Could you check a few things on this model? Use its own coordinates, in mm. Give positions to 0.01 mm unless a question says otherwise; leave off trailing zeros. Put each result on its own line as item: value.
```python
from build123d import *

# Parameters (mm, degrees)
SKETCH1_R           = 12.7
BOSS_EXTRUDE1_DEPTH = 6.35
FILLET1_R           = 1.5875
FILLET2_R           = 3.175


with BuildPart() as part:
    # Sketch1 → Boss-Extrude1 (new, symmetric)
    with BuildSketch(Plane.XY):
        Polygon((-9.43506227631135, 19.870822827505833), (-21.92616850087544, 1.7644077961790767), (-12.491106224564081, -18.10641503132676), (9.43506227631137, -19.870822827505812), (21.926168500875455, -1.764407796179048), (12.491106224564096, 18.10641503132678), align=None)
        Circle(SKETCH1_R, mode=Mode.SUBTRACT)
    extrude(amount=BOSS_EXTRUDE1_DEPTH, both=True)

    # Fillet1
    fillet1_edges = [part.edges().sort_by_distance(p)[0] for p in [
        (-17.208637362719763, -8.17100361757384, 6.35),
        (-1.5280219741263554, -18.988618929416283, 6.35),
        (15.680615388593413, -10.81761531184243, 6.35),
        (17.208637362719777, 8.171003617573865, 6.35),
        (1.5280219741263732, 18.988618929416305, 6.35),
        (17.208637362719777, 8.171003617573865, -6.35),
        (15.680615388593413, -10.81761531184243, -6.35),
        (-1.5280219741263554, -18.988618929416283, -6.35),
        (-17.208637362719763, -8.17100361757384, -6.35),
        (-15.680615388593395, 10.817615311842456, -6.35),
        (1.5280219741263732, 18.988618929416305, -6.35),
        (-15.680615388593395, 10.817615311842456, 6.35),
    ]]
    fillet(fillet1_edges, radius=FILLET1_R)

    # Fillet2
    # the kernel refuses this fillet: 3.175 mm, written as the material it takes off along each edge
    with BuildSketch(Plane(origin=(-7.862551896926124, 16.559019022921532, -6.35), x_dir=(-0.8231294167240627, 0.5678538221439602, 0), z_dir=(-0.5678538221439602, -0.8231294167240627, 0))) as fillet2_piece_1:
        with BuildLine():
            CenterArc((1.5875, -1.5875), 1.5875, 0, 90)
            Line((3.175, -1.5875), (3.175, 0))
            Line((3.175, 0), (1.5875, 0))
        make_face()
    revolve(axis=Axis((-7.862551896926124, 16.559019022921532, -6.35), (0, 0, -1)), revolution_arc=59.999999999999986, mode=Mode.SUBTRACT)
    with BuildSketch(Plane(origin=(10.409255187136749, 15.088679192772318, -6.35), x_dir=(0.08021112725072843, 0.996777896557286, 0), z_dir=(-0.996777896557286, 0.08021112725072843, 0))) as fillet2_piece_2:
        with BuildLine():
            CenterArc((1.5875, -1.5875), 1.5875, 0, 90)
            Line((3.175, -1.5875), (3.175, 0))
            Line((3.175, 0), (1.5875, 0))
        make_face()
    revolve(axis=Axis((10.409255187136749, 15.088679192772318, -6.35), (0, 0, -1)), revolution_arc=59.99999999999997, mode=Mode.SUBTRACT)
    with BuildSketch(Plane(origin=(-18.271807084062868, 1.470339830149234, -6.35), x_dir=(-0.9033405439747911, -0.4289240744133263, 0), z_dir=(0.4289240744133263, -0.9033405439747911, 0))) as fillet2_piece_3:
        with BuildLine():
            CenterArc((1.5875, -1.5875), 1.5875, 0, 90)
            Line((3.175, -1.5875), (3.175, 0))
            Line((3.175, 0), (1.5875, 0))
        make_face()
    revolve(axis=Axis((-18.271807084062868, 1.470339830149234, -6.35), (0, 0, -1)), revolution_arc=60.000000000000036, mode=Mode.SUBTRACT)
    with BuildSketch(Plane(origin=(18.27180708406288, -1.4703398301492088, -6.35), x_dir=(0.903340543974791, 0.4289240744133264, 0), z_dir=(-0.4289240744133264, 0.903340543974791, 0))) as fillet2_piece_4:
        with BuildLine():
            CenterArc((1.5875, -1.5875), 1.5875, 0, 90)
            Line((3.175, -1.5875), (3.175, 0))
            Line((3.175, 0), (1.5875, 0))
        make_face()
    revolve(axis=Axis((18.27180708406288, -1.4703398301492088, -6.35), (0, 0, -1)), revolution_arc=60.00000000000001, mode=Mode.SUBTRACT)
    with BuildSketch(Plane(origin=(-10.40925518713673, -15.0886791927723, -6.35), x_dir=(-0.0802111272507284, -0.996777896557286, 0), z_dir=(0.996777896557286, -0.0802111272507284, 0))) as fillet2_piece_5:
        with BuildLine():
            CenterArc((1.5875, -1.5875), 1.5875, 0, 90)
            Line((3.175, -1.5875), (3.175, 0))
            Line((3.175, 0), (1.5875, 0))
        make_face()
    revolve(axis=Axis((-10.40925518713673, -15.0886791927723, -6.35), (0, 0, -1)), revolution_arc=59.99999999999997, mode=Mode.SUBTRACT)
    with BuildSketch(Plane(origin=(7.862551896926148, -16.559019022921508, -6.35), x_dir=(0.823129416724063, -0.5678538221439597, 0), z_dir=(0.5678538221439597, 0.823129416724063, 0))) as fillet2_piece_6:
        with BuildLine():
            CenterArc((1.5875, -1.5875), 1.5875, 0, 90)
            Line((3.175, -1.5875), (3.175, 0))
            Line((3.175, 0), (1.5875, 0))
        make_face()
    revolve(axis=Axis((7.862551896926148, -16.559019022921508, -6.35), (0, 0, -1)), revolution_arc=60.00000000000002, mode=Mode.SUBTRACT)
    with BuildSketch(Plane(origin=(7.862551896926148, -16.559019022921508, 6.35), x_dir=(-0.0802111272507284, -0.996777896557286, 0), z_dir=(-0.996777896557286, 0.0802111272507284, 0))) as fillet2_piece_7:
        with BuildLine():
            CenterArc((1.5875, -1.5875), 1.5875, 0, 90)
            Line((3.175, -1.5875), (3.175, 0))
            Line((3.175, 0), (1.5875, 0))
        make_face()
    revolve(axis=Axis((7.862551896926148, -16.559019022921508, 6.35), (0, 0, 1)), revolution_arc=60.00000000000002, mode=Mode.SUBTRACT)
    with BuildSketch(Plane(origin=(-10.40925518713673, -15.0886791927723, 6.35), x_dir=(-0.9033405439747911, -0.4289240744133263, 0), z_dir=(-0.4289240744133263, 0.9033405439747911, 0))) as fillet2_piece_8:
        with BuildLine():
            CenterArc((1.5875, -1.5875), 1.5875, 0, 90)
            Line((3.175, -1.5875), (3.175, 0))
            Line((3.175, 0), (1.5875, 0))
        make_face()
    revolve(axis=Axis((-10.40925518713673, -15.0886791927723, 6.35), (0, 0, 1)), revolution_arc=59.99999999999997, mode=Mode.SUBTRACT)
    with BuildSketch(Plane(origin=(18.27180708406288, -1.4703398301492088, 6.35), x_dir=(0.823129416724063, -0.5678538221439597, 0), z_dir=(-0.5678538221439597, -0.823129416724063, 0))) as fillet2_piece_9:
        with BuildLine():
            CenterArc((1.5875, -1.5875), 1.5875, 0, 90)
            Line((3.175, -1.5875), (3.175, 0))
            Line((3.175, 0), (1.5875, 0))
        make_face()
    revolve(axis=Axis((18.27180708406288, -1.4703398301492088, 6.35), (0, 0, 1)), revolution_arc=60.00000000000001, mode=Mode.SUBTRACT)
    with BuildSketch(Plane(origin=(-18.271807084062868, 1.470339830149234, 6.35), x_dir=(-0.8231294167240627, 0.5678538221439602, 0), z_dir=(0.5678538221439602, 0.8231294167240627, 0))) as fillet2_piece_10:
        with BuildLine():
            CenterArc((1.5875, -1.5875), 1.5875, 0, 90)
            Line((3.175, -1.5875), (3.175, 0))
            Line((3.175, 0), (1.5875, 0))
        make_face()
    revolve(axis=Axis((-18.271807084062868, 1.470339830149234, 6.35), (0, 0, 1)), revolution_arc=60.000000000000036, mode=Mode.SUBTRACT)
    with BuildSketch(Plane(origin=(10.409255187136749, 15.088679192772318, 6.35), x_dir=(0.903340543974791, 0.4289240744133264, 0), z_dir=(0.4289240744133264, -0.903340543974791, 0))) as fillet2_piece_11:
        with BuildLine():
            CenterArc((1.5875, -1.5875), 1.5875, 0, 90)
            Line((3.175, -1.5875), (3.175, 0))
            Line((3.175, 0), (1.5875, 0))
        make_face()
    revolve(axis=Axis((10.409255187136749, 15.088679192772318, 6.35), (0, 0, 1)), revolution_arc=59.99999999999997, mode=Mode.SUBTRACT)
    with BuildSketch(Plane(origin=(-7.862551896926124, 16.559019022921532, 6.35), x_dir=(0.08021112725072843, 0.996777896557286, 0), z_dir=(0.996777896557286, -0.08021112725072843, 0))) as fillet2_piece_12:
        with BuildLine():
            CenterArc((1.5875, -1.5875), 1.5875, 0, 90)
            Line((3.175, -1.5875), (3.175, 0))
            Line((3.175, 0), (1.5875, 0))
        make_face()
    revolve(axis=Axis((-7.862551896926124, 16.559019022921532, 6.35), (0, 0, 1)), revolution_arc=59.999999999999986, mode=Mode.SUBTRACT)
    with BuildSketch(Plane(origin=(9.43506227631137, -19.870822827505812, -6.35), x_dir=(-0.9967778965572859, 0.08021112725072867, 0), z_dir=(0, 0, 1))) as fillet2_piece_13:
        with BuildLine():
            CenterArc((FILLET2_R * 0.57735026919, -FILLET2_R), FILLET2_R, 90.00000000000003, 60)
            Line((-FILLET2_R * 0.288675134595, -FILLET2_R * 0.5), (0, 0))
            Line((0, 0), (FILLET2_R * 0.57735026919, -3e-17))
        make_face()
    extrude(amount=12.7, mode=Mode.SUBTRACT)
    with BuildSketch(Plane(origin=(-12.491106224564081, -18.106415031326755, -6.35), x_dir=(-0.4289240744133256, 0.9033405439747914, 0), z_dir=(0, 0, 1))) as fillet2_piece_14:
        with BuildLine():
            CenterArc((FILLET2_R * 0.57735026919, -FILLET2_R), FILLET2_R, 90.00000000000006, 59.99999999999994)
            Line((-FILLET2_R * 0.288675134595, -FILLET2_R * 0.5), (0, 0))
            Line((0, 0), (FILLET2_R * 0.57735026919, -1.1e-16))
        make_face()
    extrude(amount=12.7, mode=Mode.SUBTRACT)
    with BuildSketch(Plane(origin=(-21.92616850087544, 1.764407796179075, -6.350000000000001), x_dir=(0.5678538221439581, 0.8231294167240641, 0), z_dir=(0, 0, 1))) as fillet2_piece_15:
        with BuildLine():
            CenterArc((FILLET2_R * 0.57735026919, -FILLET2_R), FILLET2_R, 89.99999999999986, 60.000000000000114)
            Line((-FILLET2_R * 0.288675134595, -FILLET2_R * 0.5), (0, 0))
            Line((0, 0), (FILLET2_R * 0.57735026919, 0))
        make_face()
    extrude(amount=12.700000000000001, mode=Mode.SUBTRACT)
    with BuildSketch(Plane(origin=(-9.43506227631135, 19.870822827505833, 6.35), x_dir=(-0.5678538221439603, -0.8231294167240626, 0), z_dir=(0, 0, -1))) as fillet2_piece_16:
        with BuildLine():
            CenterArc((FILLET2_R * 0.57735026919, -FILLET2_R), FILLET2_R, 89.99999999999997, 59.99999999999997)
            Line((-FILLET2_R * 0.288675134595, -FILLET2_R * 0.5), (0, 0))
            Line((0, 0), (FILLET2_R * 0.57735026919, 0))
        make_face()
    extrude(amount=12.7, mode=Mode.SUBTRACT)
    with BuildSketch(Plane(origin=(12.491106224564094, 18.10641503132678, 6.350000000000001), x_dir=(-0.9967778965572859, 0.0802111272507286, 0), z_dir=(0, 0, -1))) as fillet2_piece_17:
        with BuildLine():
            CenterArc((FILLET2_R * 0.57735026919, -FILLET2_R), FILLET2_R, 89.99999999999997, 59.99999999999994)
            Line((-FILLET2_R * 0.288675134595, -FILLET2_R * 0.5), (0, 0))
            Line((0, 0), (FILLET2_R * 0.57735026919, 0))
        make_face()
    extrude(amount=12.700000000000001, mode=Mode.SUBTRACT)
    with BuildSketch(Plane(origin=(21.926168500875455, -1.7644077961790465, 6.35), x_dir=(-0.42892407441332714, 0.9033405439747906, 0), z_dir=(0, 0, -1))) as fillet2_piece_18:
        with BuildLine():
            CenterArc((FILLET2_R * 0.57735026919, -FILLET2_R), FILLET2_R, 90.00000000000007, 59.999999999999986)
            Line((-FILLET2_R * 0.288675134595, -FILLET2_R * 0.5), (0, 0))
            Line((0, 0), (FILLET2_R * 0.57735026919, 0))
        make_face()
    extrude(amount=12.7, mode=Mode.SUBTRACT)


solid = part.part
```
1. I'm going to push flat-ended pins straight in: pin 1 (1 mm diameter, centred on y = -14, z = -3, fed in from +X); pin 2 (3 mm diameter, centred on y = 9.5, z = -1, fed in from -X); pin 3 (4 mm diameter, centred on x = -3, z = 4, fed in from +Y). Where does each tip first touch, or does it pass through?
Recorded:
pin 1: stops at x = 13.83
pin 2: stops at x = -17.62
pin 3: stops at y = 19.51
2. Thinking about a two-plate mould opening in Y: for faces 1 (the face through (-2.75, -12.4, -0.09)), 2 (the face through (-16.72, -8.08, 5.9)), 3 (the face through (-21.435, 1.748, -0.067)), which applies, pulls with the +Y half, pulls with the -Y half, needs draft (parallel to the pull), parting line crosses it, or undercut?
Recorded:
face 1: undercut
face 2: pulls with the -Y half
face 3: parting line crosses it
3. I need wall thicknesses on line 1 (Y direction, x = -3.5, z = 2.5); line 2 (Y direction, x = 0, z = -2.75); line 3 (X direction, y = 3, z = -3.75). Which ranges of each line are inside material? Lowest first, please.
Recorded:
line 1: y = -18.83 to -12.21, 12.21 to 19.39
line 2: y = -19.11 to -12.7, 12.7 to 19.11
line 3: x = -21.05 to -12.34, 12.34 to 19.66
